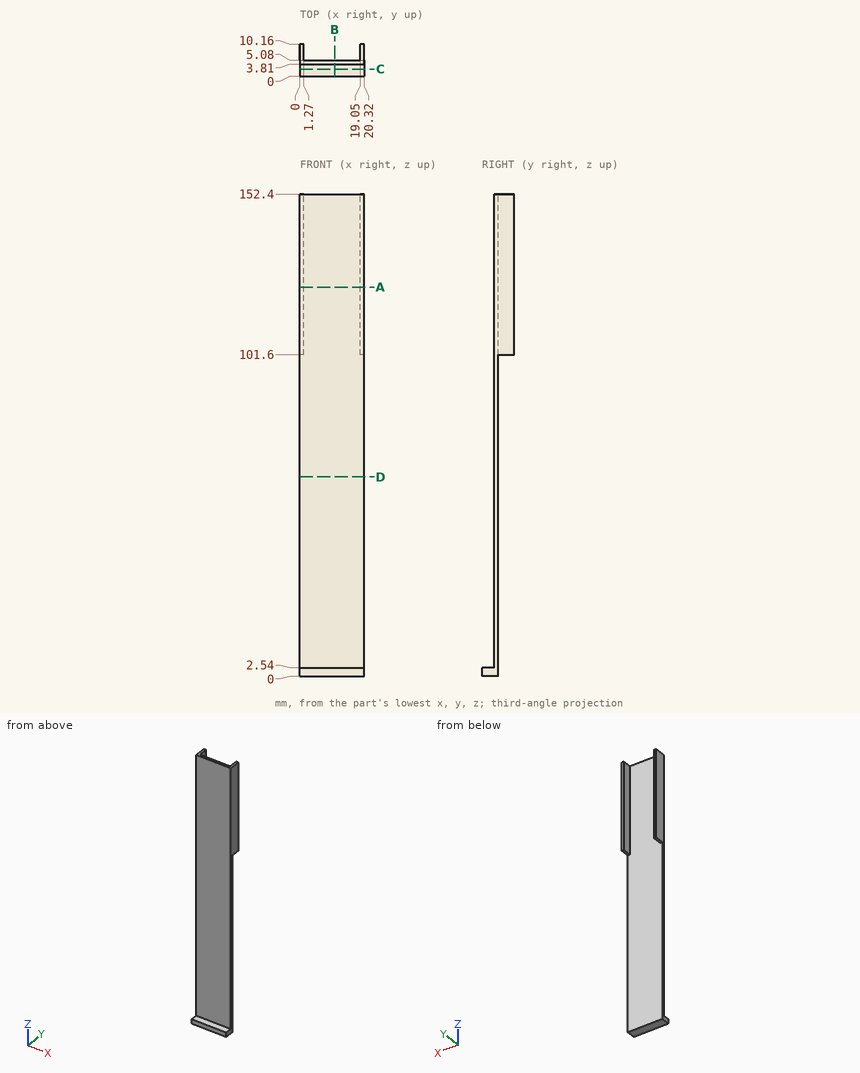
Can you work these out from the drawing? Everything is in mm from the part's minimum corner. Round coordinates to 2 decimals unless told otherwise and drop trailing zeros. Loops run counter-clockwise (first coordinate to the right, second up) from the corner with the lowest first, then second, coordinate; pieces in that order, holes last. Notation, with made-up numbers: (11, 70.25) - (50, 70.25) arc R11 ccw to (50, 74.25) - close; hole circle Ø6 at (10.25, -17). An arc over 180 degrees is marked (long way). Answer in a Markdown table with one row per item. Add a question column.
Q1. For pin 1 Ø6 at (x, z) = (7, 93.5) entering from -Y; pin 2 Ø1 at (x, y) = (0.5, 8.5) entering from -Z; pin 3 Ø3 at (x, y) = (14.5, 1.5) entering from +Z, each with a flat end and sliding along its axis, tell me the tip position at first contact or that it passes through.
Q2. I want a section at A-A on z = 123. List the corners of the cut face in (x, y) for me.
Q3. I want a section at C-C on y = 2.25. List the corners of the cut face in (x, z) for me, and give its area (3 significant figures).
Q4. I need wall thicknesses on L1, parallel to Y at x = 14.75, z = 146.5; L2, parallel to Z at x = 18, y = 2. Which ranges of each line are inside material? Lowest first, please.
Q5. I want a section at B-B on x = 11. List the corners of the cut face in (y, z) for me, and give its area (3 significant figures).
Q6. I want a section at D-D on z = 63. List the corners of the cut face in (x, y) for me, and give its area (3 significant figures).
A:
| question | item | result |
|---|---|---|
| 1 | pin 1 | y = 3.81 |
| 1 | pin 2 | z = 101.6 |
| 1 | pin 3 | z = 2.54 |
| 2 | outline | (0, 3.81) - (20.32, 3.81) - (20.32, 10.16) - (19.05, 10.16) - (19.05, 5.08) - (1.27, 5.08) - (1.27, 10.16) - (0, 10.16) - close |
| 3 | outline | (0, 0) - (20.32, 0) - (20.32, 2.54) - (0, 2.54) - close |
| 3 | area | 51.6 mm^2 |
| 4 | L1 | 3.81 to 5.08 |
| 4 | L2 | 0 to 2.54 |
| 5 | outline | (0, 0) - (5.08, 0) - (5.08, 152.4) - (3.81, 152.4) - (3.81, 2.54) - (0, 2.54) - close |
| 5 | area | 203 mm^2 |
| 6 | outline | (0, 3.81) - (20.32, 3.81) - (20.32, 5.08) - (0, 5.08) - close |
| 6 | area | 25.8 mm^2 |
